For this review, take the finished solid that the model builds, in its own axes (mm). A direction names the side the tool comes from. Give positions to 0.01 mm unless a question says otherwise; leave off trailing zeros. Loops run counter-clockwise (first coordinate to the right, second up) from the corner with the lowest first, then second, coordinate; pieces in that order, holes last. Notation, with made-up numbers: (50, -5.5) - (72, -5.5) arc R16 ccw to (72, 15.5) - close; hole circle Ø7 at (29.25, 38). An arc over 180 degrees is marked (long way). Use CSV: the item, a comma, the result in double quotes. Start each with the question number.
1. Take a section at C-C on z = 10. Give the boundary of the cut face in (x, y), plus the area to 3 significant figures.
2. Take a section at D-D on y = -19. Give the boundary of the cut face in (x, z), plus the area to 3 significant figures.
3. Wall thickness on line 1 (X direction, y = -1, z = 8.75); line 2 (Y direction, x = 14.5, z = 9.5); line 3 (X direction, y = -4.5, z = 11.75): over which ranges is each line inside the solid? List them lowest first.
4. Take a section at A-A on x = 21.5. Give the boundary of the cut face in (y, z), plus the area to 3 significant figures.
5. Take a section at B-B on y = 0. Give the boundary of the cut face in (x, z).
6. For pin 1 (3 mm diameter, centred on y = -4, z = 5, fed in from -X); pin 2 (3 mm diameter, centred on y = 19.5, z = 5.5, fed in from +X), all flat-tipped, find the tip position at first contact; note any pin that passes through.
7. For faces 4 (the cylindrical face through (-215.894, -0.559, 6.261)), 5 (the cylindrical face through (101.597, -0.279, 6.261)), list the 3-axis set-ups (+Z, -Z, +X, -X, +Y, -Y) from which the entire face can be reached by the end or side of a thin tool; tool diameter is ignored.
8. Mouldability with a two-part tool opening along X and no side actions: class faces 1 (the flat face through (31, -12.7, 6)), 2 (the cylindrical face through (114.294, 0.559, 6.261)), 3 (the flat face through (-49, -25.4, 6)) as pulls with the +X half, pulls with the -X half, needs draft (parallel to the pull), parting line crosses it, or undercut.
```python
from build123d import *

# Parameters (mm, degrees)
SKETCH1_R           = 12.7
BOSS_EXTRUDE1_DEPTH = 12.7


with BuildPart() as part:
    # Sketch1 → Boss-Extrude1 (new body)
    with BuildSketch(Plane.XY):
        with BuildLine():
            Line((-88.9, 25.4), (88.9, 25.4))
            ThreePointArc((88.9, 25.4), (114.3, 0), (88.9, -25.4))
            Line((88.9, -25.4), (-88.9, -25.4))
            Line((-88.9, -25.4), (-190.5, -25.4))
            ThreePointArc((-190.5, -25.4), (-215.9, 0), (-190.5, 25.4))
            Line((-190.5, 25.4), (-88.9, 25.4))
        make_face()
        with Locations((-88.9, 0)):
            Circle(SKETCH1_R, mode=Mode.SUBTRACT)
        with BuildLine():
            Line((88.9, 12.7), (-25.4, 12.7))
            ThreePointArc((-25.4, 12.7), (-38.1, 0), (-25.4, -12.7))
            Line((-25.4, -12.7), (88.9, -12.7))
            ThreePointArc((88.9, -12.7), (101.6, 0), (88.9, 12.7))
        make_face(mode=Mode.SUBTRACT)
    extrude(amount=BOSS_EXTRUDE1_DEPTH)


solid = part.part
```
Check result:
1,outline,"(-190.5, -25.4) - (88.9, -25.4) arc R25.4 ccw to (88.9, 25.4) - (-190.5, 25.4) arc R25.4 ccw to start; hole circle Ø25.4 at (-88.9, 0); hole (-25.4, -12.7) - (88.9, -12.7) arc R12.7 ccw to (88.9, 12.7) - (-25.4, 12.7) arc R12.7 ccw to start"
1,area,"12,300 mm²"
2,outline,"(-207.36, 0) - (105.76, 0) - (105.76, 12.7) - (-207.36, 12.7) - close"
2,area,"3,980 mm²"
3,line 1,"x = -215.88 to -101.56, -76.24 to -38.06, 101.56 to 114.28"
3,line 2,"y = -25.4 to -12.7, 12.7 to 25.4"
3,line 3,"x = -215.5 to -100.78, -77.02 to -37.28, 100.78 to 113.9"
4,outline,"(-25.4, 0) - (-12.7, 0) - (-12.7, 12.7) - (-25.4, 12.7) - close; (12.7, 0) - (25.4, 0) - (25.4, 12.7) - (12.7, 12.7) - close"
4,area,"323 mm²"
5,outline,"(-215.9, 0) - (-101.6, 0) - (-101.6, 12.7) - (-215.9, 12.7) - close; (-76.2, 0) - (-38.1, 0) - (-38.1, 12.7) - (-76.2, 12.7) - close; (101.6, 0) - (114.3, 0) - (114.3, 12.7) - (101.6, 12.7) - close"
6,pin 1,"stops at x = -215.78"
6,pin 2,"stops at x = 106.82"
7,face 4,"+Z, -Z, -X"
7,face 5,"+Z, -Z"
8,face 1,"undercut"
8,face 2,"pulls with the +X half"
8,face 3,"needs draft"
